Model file for the job. Use its own axes, mm. A direction names the side the tool comes from. Coordinates: 2 decimals unless noted, no trailing zeros. Write each loop counter-clockwise with the first axis right and the second up, starting at its lowest first coordinate (ties: lowest second). Pieces come first, ordered by that corner, then holes. Notation, with made-up numbers: (30, -24.75) -> (37, -24.75) arc R34 ccw to (37, 14.25) -> close; hole circle Ø9 at (-30, 14). An arc over 180 degrees is marked (long way). Write item = value, one per line. Start each with the question number.
from build123d import *

# Parameters (mm, degrees)
SKETCH2_W               = 88.9
SKETCH2_H               = 44.45
BOSS_EXTRUDE1_DEPTH     = 2.54
SKETCH5_W               = 83.82
SKETCH5_H               = 32.893
BOSS_EXTRUDE2_DEPTH     = 3.81
SHELL1_START            = -3.81
SHELL1_OUTLINE_W        = 81.28
SHELL1_OUTLINE_H        = 30.353
SHELL1_DEPTH            = 5.08
CUT_EXTRUDE1_DEPTH      = 51.100654936
CUT_EXTRUDE1_DEPTH_BACK = 51.100654936
SKETCH3_W               = 26.924
SKETCH3_H               = 19.558
CUT_EXTRUDE2_DEPTH      = 51.100654936
CUT_EXTRUDE2_DEPTH_BACK = 51.100654936
SKETCH4_W               = 12.446
SKETCH4_H               = 12.446
CUT_EXTRUDE3_DEPTH      = 51.100654936
CUT_EXTRUDE3_DEPTH_BACK = 2.54
SKETCH3_3_R             = 0.889
SKETCH6_W               = 14.732
SKETCH6_H               = 2.286
SKETCH6_W_2             = 15.24
SKETCH6_H_2             = 3.302
CUT_EXTRUDE4_DEPTH      = 2.54


# Read off the part's stored shape, not the designer's step: Shell1
with BuildPart() as part:
    # Sketch2 → Boss-Extrude1 (new body)
    with BuildSketch(Plane(origin=(0, 0, 0), x_dir=(1, 0, 0), z_dir=(0, 1, 0))):
        Rectangle(SKETCH2_W, SKETCH2_H)
    extrude(amount=BOSS_EXTRUDE1_DEPTH)

    # Sketch5 → Boss-Extrude2 (add)
    with BuildSketch(Plane.XZ):
        with Locations((0, 0.0635)):
            Rectangle(SKETCH5_W, SKETCH5_H)
    extrude(amount=BOSS_EXTRUDE2_DEPTH)

    # Shell1 outline → Shell1 (cut)
    with BuildSketch(Plane(origin=(0, 0, 0), x_dir=(1, 0, 0), z_dir=(0, 1, 0)).offset(SHELL1_START)):
        with Locations((0, -0.0635)):
            Rectangle(SHELL1_OUTLINE_W, SHELL1_OUTLINE_H)
    extrude(amount=SHELL1_DEPTH, mode=Mode.SUBTRACT)

    # Sketch3 → Cut-Extrude1 (cut, two sides: drawn at the far end of the back side and taken through both)
    with BuildSketch(Plane(origin=(0, 2.54, 0), x_dir=(1, 0, 0), z_dir=(0, 1, 0)).offset(-CUT_EXTRUDE1_DEPTH_BACK)):
        with Locations((25.908, 0)):
            Rectangle(SKETCH3_W, SKETCH3_H)
    extrude(amount=CUT_EXTRUDE1_DEPTH + CUT_EXTRUDE1_DEPTH_BACK, mode=Mode.SUBTRACT)

    # Sketch4 → Cut-Extrude2 (cut, two sides: drawn at the far end of the back side and taken through both)
    with BuildSketch(Plane(origin=(0, 2.54, 0), x_dir=(1, 0, 0), z_dir=(0, 1, 0)).offset(-CUT_EXTRUDE2_DEPTH_BACK)):
        with Locations((2.413, 0)):
            Rectangle(SKETCH4_W, SKETCH4_H)
        with Locations((-14.605, 0)):
            Rectangle(SKETCH4_W, SKETCH4_H)
        with Locations((-31.623, 0)):
            Rectangle(SKETCH4_W, SKETCH4_H)
    extrude(amount=CUT_EXTRUDE2_DEPTH + CUT_EXTRUDE2_DEPTH_BACK, mode=Mode.SUBTRACT)

    # Sketch3<3> → Cut-Extrude3 (cut, two sides: drawn at the far end of the back side and taken through both)
    with BuildSketch(Plane(origin=(0, 2.54, 0), x_dir=(1, 0, 0), z_dir=(0, 1, 0)).offset(-CUT_EXTRUDE3_DEPTH_BACK)):
        with Locations(Location((37.846, -12.183102804, 0), (0, 0, 90))):
            Circle(SKETCH3_3_R)
        with Locations(Location((13.97, -12.183102804, 0), (0, 0, 90))):
            Circle(SKETCH3_3_R)
        with Locations(Location((13.97, 12.217, 0), (0, 0, 90))):
            Circle(SKETCH3_3_R)
        with Locations(Location((37.846, 12.183102804, 0), (0, 0, 90))):
            Circle(SKETCH3_3_R)
    extrude(amount=CUT_EXTRUDE3_DEPTH + CUT_EXTRUDE3_DEPTH_BACK, mode=Mode.SUBTRACT)

    # Sketch6 → Cut-Extrude4 (cut)
    with BuildSketch(Plane(origin=(0, 2.54, 0), x_dir=(1, 0, 0), z_dir=(0, 1, 0))):
        with Locations((25.908, -10.922)):
            Rectangle(SKETCH6_W, SKETCH6_H)
        with Locations((25.908, 11.43)):
            Rectangle(SKETCH6_W_2, SKETCH6_H_2)
    extrude(amount=-CUT_EXTRUDE4_DEPTH, mode=Mode.SUBTRACT)


solid = part.part
(1) Mould opens along X. For faces 5 (the face through (41.91, -2, 0)), 6 (the face through (-41.91, -2, 0)), 7 (the face through (-1, -1, 15.24)) say: released by +X, released by -X, zero draft, split by the parting line, or undercut.
(2) Drill centre lines: line 1 along X through (y, z) = (2, 5.5); line 2 along Z through (x, y) = (22, -0.5); line 3 along X through (y, z) = (-2, -12.5). Where is each one in solid material? Low to high.
(3) Saw through at A-A (z = -3). Give the cut face in (x, y), then the cut area to 3 significant figures.
(4) Saw through at B-B (x = 13.97). Give the cut face in (y, z) (3 decimals), then the cut area to 3 significant figures.
(5) Saw through at D-D (x = 4). Give the cut face in (y, z) (3 decimals), then the cut area to 3 significant figures.
(6) 3-axis set-ups, long thin cutter, end or side, ignore diameter. For faces 1 (the face through (38.635, 1.896, -12.593)), 2 (the face through (-1, -2, -16.383)), 3 (the face through (-10, 1.27, -7)), 4 (the face through (-1, -2, 16.51)): which of +Z, -Z, +X, -X, +Y, -Y reach the whole face in a straight line?
(7) Drop flat-ended pins along their axis: pin 1 Ø1.1 at (y, z) = (-2, 1.5) entering from -X; pin 2 Ø3 at (x, z) = (37.85, 12.18) entering from -Y; pin 3 Ø1 at (x, y) = (-15.5, -1.5) entering from -Z. Give the stop position or say it passes through.
(8) Saw through at C-C (z = 8.5). Give the cut face in (x, y), then the cut area to 3 significant figures.
Returned:
q1.face_5 = released by +X
q1.face_6 = released by -X
q1.face_7 = undercut
q2.line_1 = -44.45 to -37.85, -25.4 to -20.83, -8.38 to -3.81, 8.64 to 12.45, 39.37 to 44.45
q2.line_2 = -16.38 to -15.11, 15.24 to 16.51
q2.line_3 = -41.91 to -40.64, 40.64 to 41.91
q3.outline = (-44.45, 0) -> (-41.91, 0) -> (-41.91, -3.81) -> (-40.64, -3.81) -> (-40.64, 1.27) -> (-37.85, 1.27) -> (-37.85, 2.54) -> (-44.45, 2.54) -> close; (-25.4, 1.27) -> (-20.83, 1.27) -> (-20.83, 2.54) -> (-25.4, 2.54) -> close; (-8.38, 1.27) -> (-3.81, 1.27) -> (-3.81, 2.54) -> (-8.38, 2.54) -> close; (8.64, 1.27) -> (12.45, 1.27) -> (12.45, 2.54) -> (8.64, 2.54) -> close; (39.37, 1.27) -> (40.64, 1.27) -> (40.64, -3.81) -> (41.91, -3.81) -> (41.91, 0) -> (44.45, 0) -> (44.45, 2.54) -> (39.37, 2.54) -> close
q3.area = 50.6 mm2
q4.outline = (-3.81, -16.383) -> (0, -16.383) -> (0, -22.225) -> (2.54, -22.225) -> (2.54, -13.106) -> (1.27, -13.106) -> (1.27, -15.113) -> (-3.81, -15.113) -> close; (-3.81, 15.24) -> (1.27, 15.24) -> (1.27, 13.072) -> (2.54, 13.072) -> (2.54, 22.225) -> (0, 22.225) -> (0, 16.51) -> (-3.81, 16.51) -> close; (1.27, -11.328) -> (2.54, -11.328) -> (2.54, -9.779) -> (1.27, -9.779) -> close; (1.27, 9.779) -> (2.54, 9.779) -> (2.54, 11.294) -> (1.27, 11.294) -> close
q4.area = 54.7 mm2
q5.outline = (-3.81, -16.383) -> (0, -16.383) -> (0, -22.225) -> (2.54, -22.225) -> (2.54, -6.223) -> (1.27, -6.223) -> (1.27, -15.113) -> (-3.81, -15.113) -> close; (-3.81, 15.24) -> (1.27, 15.24) -> (1.27, 6.223) -> (2.54, 6.223) -> (2.54, 22.225) -> (0, 22.225) -> (0, 16.51) -> (-3.81, 16.51) -> close
q5.area = 68.2 mm2
q6.face_1 = +Y, -Y
q6.face_2 = -Z, +X, -X, -Y
q6.face_3 = -Y
q6.face_4 = +Z, +X, -X, -Y
q7.pin_1 = -41.91
q7.pin_2 = 1.27
q7.pin_3 = -16.38
q8.outline = (-44.45, 0) -> (-41.91, 0) -> (-41.91, -3.81) -> (-40.64, -3.81) -> (-40.64, 1.27) -> (12.45, 1.27) -> (12.45, 2.54) -> (-44.45, 2.54) -> close; (39.37, 1.27) -> (40.64, 1.27) -> (40.64, -3.81) -> (41.91, -3.81) -> (41.91, 0) -> (44.45, 0) -> (44.45, 2.54) -> (39.37, 2.54) -> close
q8.area = 98.1 mm2
